Can you work these out from the drawing? Everything is in mm from the part's minimum corner. A direction names the side the tool comes from. Give positions to 0.01 mm unless a question says otherwise; leave off trailing zeros. Order: outer loops, then holes, each group sorted by start corner. A loop starts at its lowest first (then second) coordinate and runs counter-clockwise, first axis right, second up. Notation, with made-up numbers: (46, 1.25) -> (90, 1.25) arc R13 cw to (90, 17.25) -> close; hole circle Ø9 at (80.25, 37). An arc over 180 degrees is marked (long way). One line per item, written item: value.
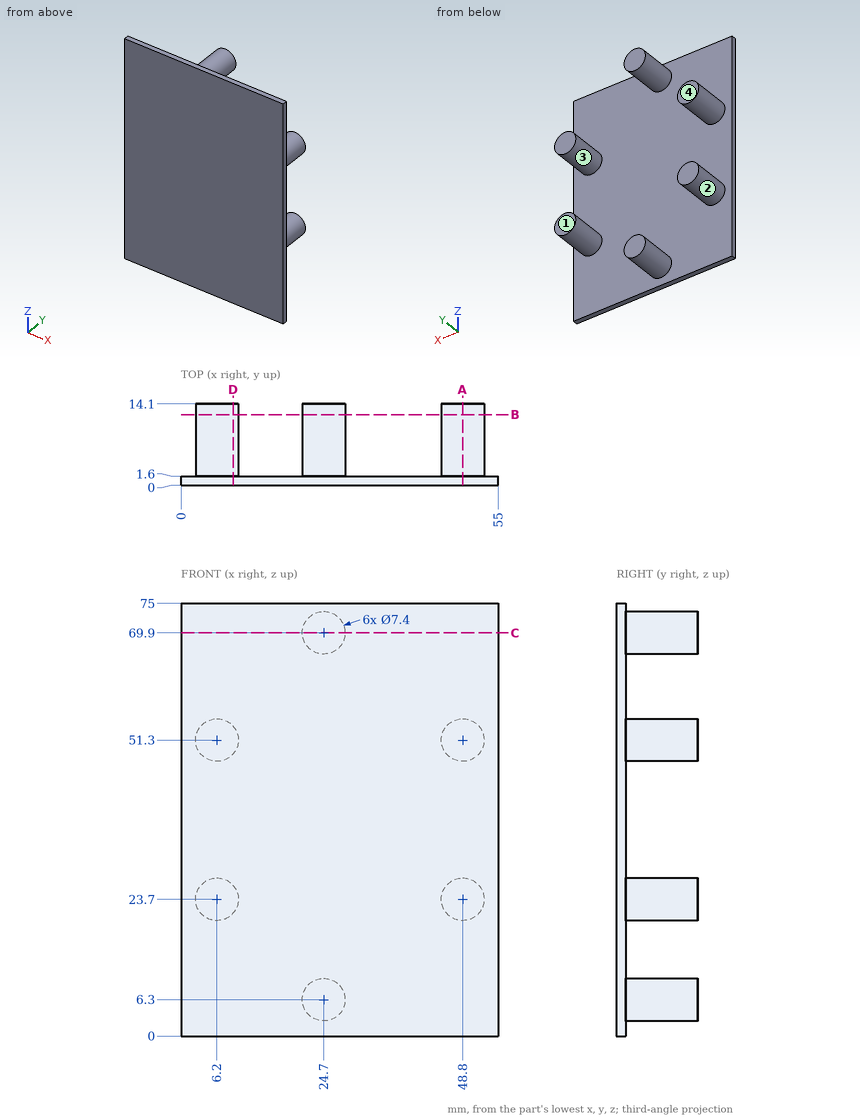
1) For the marked faces 3 and 4, which set-ups out of +Z, -Z, +X, -X, +Y, -Y let a thin tool reach every point of the face, with its end or its side?
Answer below:
face 3: +Y
face 4: +Z, -Z, +X, -X, +Y
2) We'd pull the mould along Z, two halves only. Please class the marked faces 1 and 2: +Z half, -Z half, draft (parallel to the pull), parting line (faces both ways), or undercut.
Answer below:
face 1: draft
face 2: undercut
3) For P1, Ø4, axis at x = 48.5, y = 7, coming from the +Z side; P2, Ø8, axis at x = 42.5, z = 12.5, coming from the +Y side; P3, Ø4, axis at y = 10.5, z = 18.5, coming from the +X side, each with a flat end and sliding along its axis, tell me the tip position at first contact or that it passes through.
Answer below:
P1: stops at z = 55
P2: stops at y = 1.6
P3: stops at x = 50.66
4) Suppose I cut it at B-B, the plane y = 12.25. Write out the boundary of the cut face in (x, z).
Answer below:
outline: circle Ø7.4 at (6.2, 23.7); circle Ø7.4 at (6.2, 51.3); circle Ø7.4 at (24.7, 6.3); circle Ø7.4 at (24.7, 69.9); circle Ø7.4 at (48.8, 23.7); circle Ø7.4 at (48.8, 51.3)
5) Suppose I cut it at D-D, the plane x = 9. Write out the boundary of the cut face in (y, z).
Answer below:
outline: (0, 0) -> (1.6, 0) -> (1.6, 21.28) -> (14.1, 21.28) -> (14.1, 26.12) -> (1.6, 26.12) -> (1.6, 48.88) -> (14.1, 48.88) -> (14.1, 53.72) -> (1.6, 53.72) -> (1.6, 75) -> (0, 75) -> close
6) Suppose I cut it at C-C, the plane z = 69.9. Write out the boundary of the cut face in (x, y).
Answer below:
outline: (0, 0) -> (55, 0) -> (55, 1.6) -> (28.4, 1.6) -> (28.4, 14.1) -> (21, 14.1) -> (21, 1.6) -> (0, 1.6) -> close
7) If I drill on line 1 along Y through (x, z) = (46.5, 30); line 2 along X through (y, z) = (9.5, 70); line 3 along X through (y, z) = (5.25, 50), over which ranges is the centre line in solid material (lowest first)?
Answer below:
line 1: y = 0 to 1.6
line 2: x = 21 to 28.4
line 3: x = 2.74 to 9.66, 45.34 to 52.26
8) Suppose I cut it at A-A, the plane x = 48.8. Write out the boundary of the cut face in (y, z), then the cut area to 3 significant figures.
Answer below:
outline: (0, 0) -> (1.6, 0) -> (1.6, 20) -> (14.1, 20) -> (14.1, 27.4) -> (1.6, 27.4) -> (1.6, 47.6) -> (14.1, 47.6) -> (14.1, 55) -> (1.6, 55) -> (1.6, 75) -> (0, 75) -> close
area: 305 mm2
